Input: part model. Units: mm. Frame: model coordinates. Face numbers are marked on the shaded views. Coordinates: 2 decimals unless noted, no trailing zeros. Order: outer loops, then holes, each group sorted by start corner. A loop starts at its lowest first (then second) coordinate and runs counter-clockwise, first axis right, second up. Notation, with made-up numbers: M 11.25,-28.5 L 68.25,-28.5 A22 cw 68.25,-3.5 Z; hole C 17.5,-6.5 d10. An arc over 180 degrees is marked long. Answer in a Markdown table with one row per item.
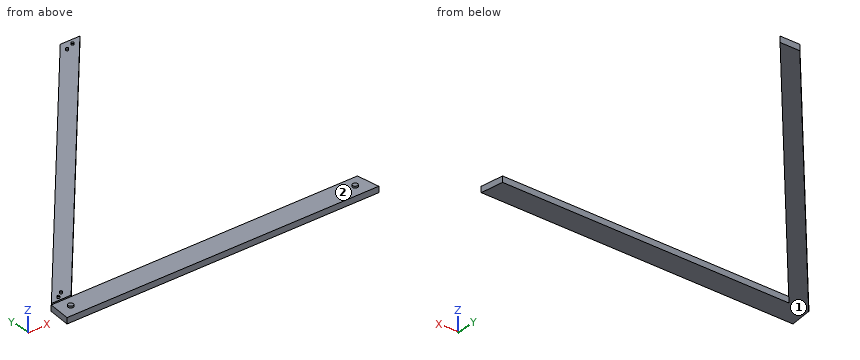
from build123d import *

# Parameters (mm, degrees)
F1_DEPTH = 0.889
F3_DEPTH = 0.381
F4_R     = 0.1778
F4_R_2   = 0.381
F5_DEPTH = 0.254
F7_DEPTH = 25.4


with BuildPart() as f1:
    # F0 (on Top) → F1 (new body)
    with BuildSketch(Plane.XY):
        Polygon((-24.947381, -12.216053), (-26.81388, -12.216053), (-26.81388, -15.690773), (23.98612, -15.690773), (23.98612, -12.216053), (-21.899363, -12.216053), (17.63612, 34.014853), (14.588101, 34.014853), align=None)
    extrude(amount=F1_DEPTH)

    # F2 (on face) → F3 (cut)
    with BuildSketch(Plane.XY.offset(0.889)):
        Polygon((-24.730167, -11.962053), (-24.947381, -12.216053), (-21.899363, -12.216053), (-21.682148, -11.962053), align=None)
    extrude(amount=-F3_DEPTH, mode=Mode.SUBTRACT)

    # F4 (on face) → F5 (join)
    with BuildSketch(Plane.XY.offset(0.889)):
        with Locations((-23.253968, -11.468455)):
            Circle(F4_R)
        with Locations((-22.337059, -10.852045)):
            Circle(F4_R)
        with Locations((-23.38488, -13.950873)):
            Circle(F4_R_2)
        with Locations((15.699644, 33.05497)):
            Circle(F4_R)
        with Locations((14.366657, 32.453973)):
            Circle(F4_R)
        with Locations((20.55712, -13.938173)):
            Circle(F4_R_2)
    extrude(amount=F5_DEPTH)

    # F6 (on face) → F7 (cut)
    with BuildSketch(Plane.XY.offset(0.889)):
        Polygon((-25.387098, -15.690773), (-24.960456, -12.216053), (-26.81388, -12.216053), (-26.81388, -15.690773), align=None)
        Polygon((22.33512, -12.216053), (22.761762, -15.690773), (23.98612, -15.690773), (23.98612, -12.216053), align=None)
    extrude(amount=-F7_DEPTH, mode=Mode.SUBTRACT)


solid = f1.part
1) Material intervals for probe 1 along Z at (x, y) = (-3.5, 12.5); probe 2 along Y at (x, z) = (18, 0.5); probe 3 along Y at (x, z) = (-21, 0.1), sorted ascending.
Resolved:
| item | result |
|---|---|
| probe 1 | z = 0 to 0.89 |
| probe 2 | y = -15.69 to -12.22 |
| probe 3 | y = -15.69 to -12.22, -11.16 to -7.6 |
2) Cut plane D-D, the plane x = 18.5. Output: boundary loops of the cut face in (y, z), and give its area (3 significant figures).
Resolved:
| item | result |
|---|---|
| outline | M -15.69,0 L -12.22,0 L -12.22,0.89 L -15.69,0.89 Z |
| area | 3.09 mm2 |
3) Cut plane C-C, the plane y = 21.5. Output: boundary loops of the cut face in (x, z), and give its area (3 significant figures).
Resolved:
| item | result |
|---|---|
| outline | M 3.89,0 L 6.93,0 L 6.93,0.89 L 3.89,0.89 Z |
| area | 2.71 mm2 |
4) Cut plane B-B, the plane x = -8. Output: boundary loops of the cut face in (y, z), and give its area (3 significant figures).
Resolved:
| item | result |
|---|---|
| outline | M -15.69,0 L -12.22,0 L -12.22,0.89 L -15.69,0.89 Z; M 4.04,0 L 7.6,0 L 7.6,0.89 L 4.04,0.89 Z |
| area | 6.26 mm2 |
5) Contact query for a flat-ended pin moving along its axis: pin 1 (3 mm diameter, centred on x = -3, y = -13.5, fed in from +Z). Output: stop coordinate, or through.
Resolved:
| item | result |
|---|---|
| pin 1 | stops at z = 0.89 |
6) Mould query, pull axis X, two halves, no side actions, for the marked faces 1 and 2. Classes: +X half, -X half, draft (parallel to the pull), parting line (faces both ways), or undercut.
Resolved:
| item | result |
|---|---|
| face 1 | draft |
| face 2 | undercut |
